```python
from build123d import *

# Parameters (mm, degrees)
F1_DEPTH = 10
F2_W     = 5
F2_H     = 10
F3_DEPTH = 2


with BuildPart() as f1:
    # F0 (on Top) → F1 (new body, symmetric)
    with BuildSketch(Plane.XY):
        with BuildLine():
            Line((21.1354362127, 15.4197925036), (0, 15.4197925036))
            Line((0, 15.4197925036), (0, 12.9197925036))
            Line((0, 12.9197925036), (20.1995696905, 12.9197925036))
            ThreePointArc((20.1995696905, 12.9197925036), (20.4570887279, 12.8483761539), (20.6410434869, 12.654528285))
            Line((20.6410434869, 12.654528285), (26.7597329087, 1.1469471563))
            ThreePointArc((26.7597329087, 1.1469471563), (26.7571548794, 1.0484961925), (26.6714381494, 1))
            Line((26.6714381494, 1), (25.3378660976, 1))
            Line((25.3378660976, 1), (25.3378660976, 0))
            Line((25.3378660976, 0), (28.4966643127, 0))
            ThreePointArc((28.4966643127, 0), (28.8502177032, 0.1464466094), (28.9966643127, 0.5))
            Line((28.9966643127, 0.5), (28.9966643127, 0.7512095949))
            ThreePointArc((28.9966643127, 0.7512095949), (28.94319662, 1.186669007), (28.7859699798, 1.5962584079))
            Line((28.7859699798, 1.5962584079), (21.5769100091, 15.154528285))
            ThreePointArc((21.5769100091, 15.154528285), (21.3929552502, 15.3483761539), (21.1354362127, 15.4197925036))
        make_face()
    extrude(amount=F1_DEPTH, both=True)

    # F2 (on face) → F3 (cut)
    with BuildSketch(Plane.XZ.offset(-12.9197925036)):
        with Locations((2.5, 0)):
            Rectangle(F2_W, F2_H)
    extrude(amount=-F3_DEPTH, mode=Mode.SUBTRACT)

    # F4: F1 across plane


with BuildPart() as f1_1:
    add(f1.part)
    add(f1.part.mirror(Plane.YZ))


solid = f1_1.part
```
Design review of the part built by this model. Coordinates are the model's own, in mm. A direction names the side the tool comes from. Round coordinates to 2 decimals unless told otherwise and drop trailing zeros. Write each loop counter-clockwise with the first axis right and the second up, starting at its lowest first coordinate (ties: lowest second). Pieces come first, ordered by that corner, then holes.
Item 1: We need section B-B on y = 14. Write out the cut boundary in (x, z).
Item 2: We need section D-D on y = 3. Write out the cut boundary in (x, z), and give its area (3 significant figures).
Item 3: The part is to be moulded in two halves that separate along Y. For faces 6 (the flat face through (-5, 14, 0)), 7 (the flat face through (27, 0, 0)), 8 (the flat face through (-23.66, 6.98, 0.14)), say which applies: +Y half, -Y half, draft (parallel to the pull), parting line (faces both ways), or undercut.
Item 4: Clearance check with flat-ended pins moving along their axes: pin 1 Ø1.6 at (y, z) = (13.5, 2.5) entering from +X; pin 2 Ø8 at (x, z) = (2, 0.5) entering from -Y; pin 3 Ø1.1 at (x, z) = (25.5, 4) entering from +Y; pin 4 Ø5 at (y, z) = (1.5, 6.5) entering from +X. State where each tip first meets the part, or that it passes through.
Item 5: We need section C-C on x = 2.5. Write out the cut boundary in (y, z), and give its area (3 significant figures).
Item 6: For faces 1 (the flat face through (26, 1, 0)), 2 (the flat face through (0, 14, 5)), 3 (the flat face through (0, 14, -10)), 4 (the flat face through (25.338, 0.5, 0.1)), 5 (the flat face through (25.23, 8.28, 0.14)), list the 3-axis set-ups (+Z, -Z, +X, -X, +Y, -Y) from which the entire face can be reached by the end or side of a thin tool; tool diameter is ignored.
Item 7: We need section A-A on z = -2. Write out the cut boundary in (x, y), and give its area (3 significant figures).
Item 8: For probe 1 along Y at (x, z) = (-19, -5.5); probe 2 along X at (y, z) = (13.75, 0.25); probe 3 along X at (y, z) = (4, -6), list the stretches that pass through material, from the lowest coordinate up.
Returned:
1. outline: (-22.19, -10) - (22.19, -10) - (22.19, 10) - (-22.19, 10) - close; hole (-5, -5) - (5, -5) - (5, 5) - (-5, 5) - close
2. outline: (-28.04, -10) - (-25.77, -10) - (-25.77, 10) - (-28.04, 10) - close; (25.77, -10) - (28.04, -10) - (28.04, 10) - (25.77, 10) - close
2. area: 90.6 mm2
3. face 6: draft
3. face 7: -Y half
3. face 8: undercut
4. pin 1: stops at x = 22.88
4. pin 2: stops at y = 12.92
4. pin 3: stops at y = 8.81
4. pin 4: stops at x = 29
5. outline: (12.92, -10) - (15.42, -10) - (15.42, 10) - (12.92, 10) - (12.92, 5) - (14.92, 5) - (14.92, -5) - (12.92, -5) - close
5. area: 30.0 mm2
6. face 1: +Z, -Z
6. face 2: -Y
6. face 3: -Z, +X, -X, +Y, -Y
6. face 4: +Z, -Z, -Y
6. face 5: +Z, -Z, +X, +Y
7. outline: (-29, 0.5) arc R0.5 ccw to (-28.5, 0) - (-25.34, 0) - (-25.34, 1) - (-26.67, 1) arc R0.1 cw to (-26.76, 1.15) - (-20.64, 12.65) arc R0.5 cw to (-20.2, 12.92) - (-5, 12.92) - (-5, 14.92) - (5, 14.92) - (5, 12.92) - (20.2, 12.92) arc R0.5 cw to (20.64, 12.65) - (26.76, 1.15) arc R0.1 cw to (26.67, 1) - (25.34, 1) - (25.34, 0) - (28.5, 0) arc R0.5 ccw to (29, 0.5) - (29, 0.75) arc R1.8 ccw to (28.79, 1.6) - (21.58, 15.15) arc R0.5 ccw to (21.14, 15.42) - (-21.14, 15.42) arc R0.5 ccw to (-21.58, 15.15) - (-28.79, 1.6) arc R1.8 ccw to (-29, 0.75) - close
7. area: 152 mm2
8. probe 1: y = 12.92 to 15.42
8. probe 2: x = -22.32 to -5, 5 to 22.32
8. probe 3: x = -27.51 to -25.24, 25.24 to 27.51
